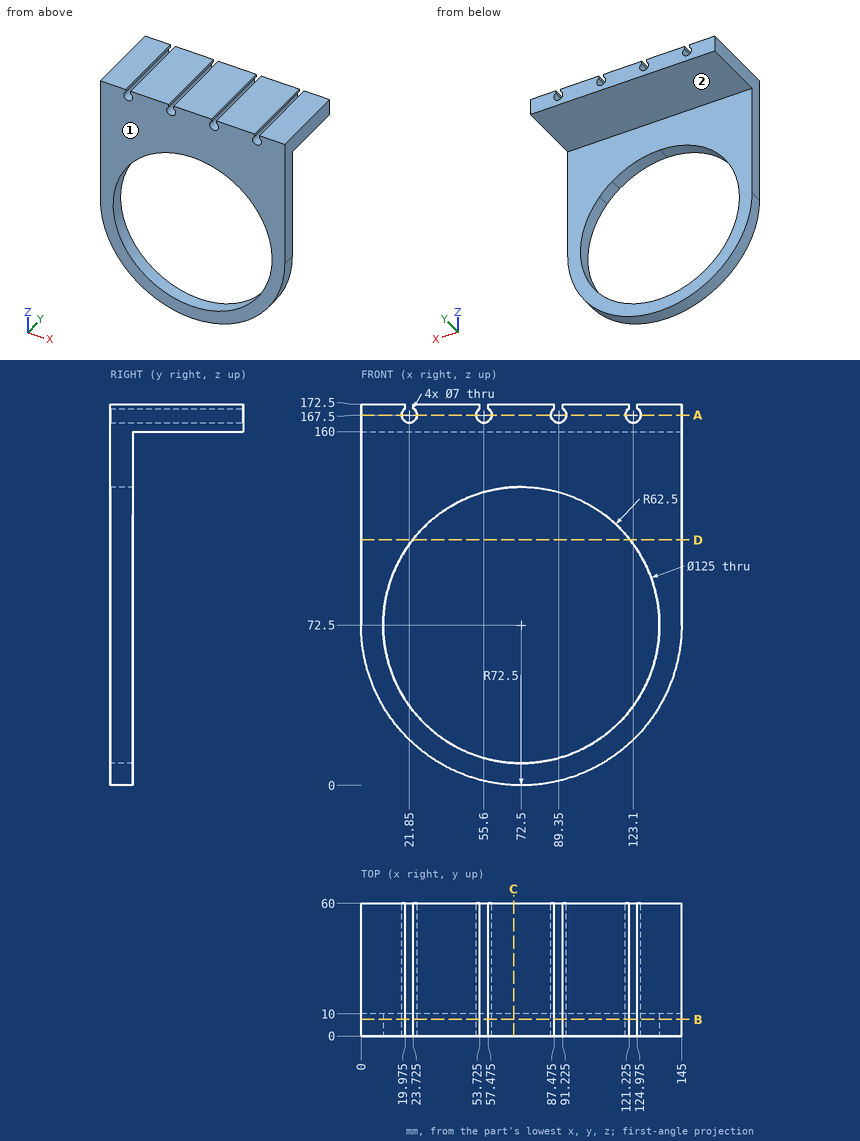
Geometry check sheet. Reference: drawing and pictorial views, mm from the part's lowest x, y, z. A direction names the side the tool comes from. Give positions to 0.01 mm unless a question says otherwise; leave off trailing zeros. Loops run counter-clockwise (first coordinate to the right, second up) from the corner with the lowest first, then second, coordinate; pieces in that order, holes last. Notation, with made-up numbers: M -23,89 L -18,89 A32 cw -18,125 Z; hole C 10,52.5 d9. An arc over 180 degrees is marked long. Use a Markdown table: item, result. Add a question column.
Q1. Sectioned sample at B-B, the plane y = 7.5. Record the cut outline in (x, z) (3 decimals), then the cut area to 3 significant figures.
Q2. Go/stop test with flat-tipped pins: pin 1 (8 mm diameter, centred on x = 55.6, z = 167.5, fed in from -Y); pin 2 (12 mm diameter, centred on x = 90, y = 38, fed in from -Z); pin 3 (10 mm diameter, centred on x = 100.5, y = 9, fed in from -Z) (3 decimals). Record where each tip stops, or that it passes through.
Q3. Sectioned sample at D-D, the plane z = 111. Record the cut outline in (x, y).
Q4. Sectioned sample at A-A, the plane z = 167.5. Record the cut outline in (x, y), then the cut area to 3 significant figures.
Q5. Scan lines: line 1 along X through (y, z) = (45.5, 167.5); line 2 along X through (y, z) = (7, 72); line 3 along Z through (x, y) = (68, 26). Record each from-to range of solid material in increasing order. Write a range as [from, to].
Q6. Sectioned sample at C-C, the plane x = 69. Record the cut outline in (y, z).
Q7. Tool access check on the marked faces 1 and 2. Record the directions out of +Z, -Z, +X, -X, +Y, -Y that give a thin tool (end or side, any length) a straight path to the whole face; none if there is none.
Verdict:
| question | item | result |
|---|---|---|
| 1 | outline | M 0,72.5 A72.5 ccw 145,72.5 L 145,172.5 L 124.975,172.5 L 124.975,170.455 A3.5 cw long 121.225,170.455 L 121.225,172.5 L 91.225,172.5 L 91.225,170.455 A3.5 cw long 87.475,170.455 L 87.475,172.5 L 57.475,172.5 L 57.475,170.455 A3.5 cw long 53.725,170.455 L 53.725,172.5 L 23.725,172.5 L 23.725,170.455 A3.5 cw long 19.975,170.455 L 19.975,172.5 L 0,172.5 Z; hole C 72.5,72.5 d125 |
| 1 | area | 10,300 mm^2 |
| 2 | pin 1 | y = 0 |
| 2 | pin 2 | z = 160 |
| 2 | pin 3 | z = 3.745 |
| 3 | outline | M 0,0 L 23.27,0 L 23.27,10 L 0,10 Z; M 121.73,0 L 145,0 L 145,10 L 121.73,10 Z |
| 4 | outline | M 0,0 L 18.35,0 L 18.35,60 L 0,60 Z; M 25.35,0 L 52.1,0 L 52.1,60 L 25.35,60 Z; M 59.1,0 L 85.85,0 L 85.85,60 L 59.1,60 Z; M 92.85,0 L 119.6,0 L 119.6,60 L 92.85,60 Z; M 126.6,0 L 145,0 L 145,60 L 126.6,60 Z |
| 4 | area | 7,020 mm^2 |
| 5 | line 1 | [0, 18.35], [25.35, 52.1], [59.1, 85.85], [92.85, 119.6], [126.6, 145] |
| 5 | line 2 | [0, 10], [135, 145] |
| 5 | line 3 | [160, 172.5] |
| 6 | outline | M 0,0.08 L 10,0.08 L 10,10.1 L 0,10.1 Z; M 0,134.9 L 10,134.9 L 10,160 L 60,160 L 60,172.5 L 0,172.5 Z |
| 7 | face 1 | +Z, -Z, +X, -X, -Y |
| 7 | face 2 | -Z, +X, -X, +Y |
